Geometry: final body of the model. Coordinates: model frame, mm. A direction names the side the tool comes from. Give positions to 0.01 mm unless a question says otherwise; leave off trailing zeros. Order: outer loops, then holes, each group sorted by start corner. A loop starts at its lowest first (then second) coordinate and runs counter-clockwise, first axis right, second up. Notation, with made-up numbers: (75, -39) -> (127, -39) arc R34 cw to (127, -1) -> close; hole circle Ø11 at (30, 24). An arc over 180 degrees is marked (long way). Answer in a Markdown table with one row per item. Add a question column.
Q1. Cut plane B-B on z = -2.45. Return the cut outline in (x, y).
Q2. Set-up query: faces 5 (the face through (-1.9, 0.1, -1)), 6 (the face through (2, 0, -1.9)), 7 (the face through (-2, 0, -1.9)). Return all of +Z, -Z, +X, -X, +Y, -Y with unobstructed straight access to the full face (end or side cutting, diameter ignored); none if empty.
Q3. Pull-direction query (Y, two-part tool) for faces 1 (the face through (0.04, -4.75, -1.38)), 2 (the face through (0, 3, 0)), 3 (the face through (-0.04, 4.75, -1.38)), 4 (the face through (-1.23, 0.05, -1.38)); classes: +Y half, -Y half, draft (parallel to the pull), parting line (faces both ways), or undercut.
Q4. Cut plane C-C on y = 0. Return the cut outline in (x, z), and give its area (3 significant figures).
Q5. Cut plane A-A on x = 0. Return the cut outline in (y, z), and give its area (3 significant figures).
Q6. Contact query for flat-ended pins moving along their axis: P1, Ø1.5, axis at x = 1, z = -2, coming from the +Y side; P2, Ø0.7, axis at x = -2, y = 1, coming from the -Z side; P3, Ø1.5, axis at x = -2, z = -1.5, coming from the +Y side. Output: stop coordinate, or through.
Q7. Cut plane D-D on y = 2. Return the cut outline in (x, z).
Q8. Line query: line 1 along Y through (x, z) = (0, -0.55); line 2 along X through (y, z) = (0, -2.2); line 3 along Y through (x, z) = (-1.1, -1.6). Output: solid intervals per line, ascending. Write a range as from..to.
from build123d import *

# Parameters (mm, degrees)
BOSS_EXTRU_1_DEPTH      = 4.75
ESQUISSE1_OUTSIDE_W     = 9.876
ESQUISSE1_OUTSIDE_H     = 13.776
ENL_V_MAT_EXTRU_1_DEPTH = 7.18405207
TROU_TARAUD_M31_D       = 2.45875


with BuildPart() as part:
    # Esquisse2 → Boss.-Extru.1 (new, symmetric)
    with BuildSketch(Plane(origin=(0, 0, 0), x_dir=(1, 0, 0), z_dir=(0, 1, 0))):
        Polygon((0.9, 0), (2.8, 1.9), (1.45, 1.9), (1.45, 2.8), (-1.45, 2.8), (-1.45, 1.9), (-2.8, 1.9), (-0.9, 0), align=None)
    extrude(amount=BOSS_EXTRU_1_DEPTH, both=True)

    # Esquisse1 outside → Enlèv. mat.-Extru.1 (cut, through all)
    with BuildSketch(Plane.XY):
        Rectangle(ESQUISSE1_OUTSIDE_W, ESQUISSE1_OUTSIDE_H)
        with BuildLine():
            Line((-2.8, -3.581739419), (-2.8, 3.581739419))
            ThreePointArc((-2.8, 3.581739419), (0, 4.75), (2.8, 3.581739419))
            Line((2.8, 3.581739419), (2.8, -3.581739419))
            ThreePointArc((2.8, -3.581739419), (0, -4.75), (-2.8, -3.581739419))
        make_face(mode=Mode.SUBTRACT)
    extrude(amount=-ENL_V_MAT_EXTRU_1_DEPTH, mode=Mode.SUBTRACT)

    # Trou taraudé M31 (through all)
    with Locations(Plane(origin=(0, 0, -2.8), x_dir=(-1, 0, 0), z_dir=(0, 0, -1))):
        with Locations((0, 0)):
            Hole(TROU_TARAUD_M31_D / 2)


solid = part.part
Completed:
| question | item | result |
|---|---|---|
| 1 | outline | (-1.45, -4.47) arc R3.94 ccw to (1.45, -4.47) -> (1.45, 4.47) arc R3.94 ccw to (-1.45, 4.47) -> close; hole circle Ø2.46 at (0, 0) |
| 2 | face 5 | +Z, -X, +Y, -Y |
| 2 | face 6 | -Z, +X, +Y, -Y |
| 2 | face 7 | -Z, -X, +Y, -Y |
| 3 | face 1 | -Y half |
| 3 | face 2 | draft |
| 3 | face 3 | +Y half |
| 3 | face 4 | undercut |
| 4 | outline | (-2.8, -1.9) -> (-1.45, -1.9) -> (-1.45, -2.8) -> (-1.23, -2.8) -> (-1.23, -0.33) -> close; (1.23, -2.8) -> (1.45, -2.8) -> (1.45, -1.9) -> (2.8, -1.9) -> (1.23, -0.33) -> close |
| 4 | area | 2.86 mm² |
| 5 | outline | (-4.75, -2.8) -> (-1.23, -2.8) -> (-1.23, 0) -> (-4.75, 0) -> close; (1.23, -2.8) -> (4.75, -2.8) -> (4.75, 0) -> (1.23, 0) -> close |
| 5 | area | 19.7 mm² |
| 6 | P1 | stops at y = 4.74 |
| 6 | P2 | stops at z = -1.9 |
| 6 | P3 | stops at y = 4.55 |
| 7 | outline | (-2.8, -1.9) -> (-1.45, -1.9) -> (-1.45, -2.8) -> (1.45, -2.8) -> (1.45, -1.9) -> (2.8, -1.9) -> (0.9, 0) -> (-0.9, 0) -> close |
| 8 | line 1 | y = -4.75..-1.23, 1.23..4.75 |
| 8 | line 2 | x = -1.45..-1.23, 1.23..1.45 |
| 8 | line 3 | y = -4.59..-0.55, 0.55..4.59 |
